Drawing for the job (mm, zero at the part's lowest x, y, z). Coordinates: 2 decimals unless noted, no trailing zeros. Write each loop counter-clockwise with the first axis right and the second up, starting at its lowest first coordinate (ties: lowest second). Pieces come first, ordered by that corner, then holes. Notation, with made-up numbers: M -14.5,-31 L 14.5,-31 A34 ccw 14.5,-1 Z; hole C 89,-5 d1. An arc over 180 degrees is marked long. Use a Markdown table: item, result. Add a question column.
Q1. Wall check: L1, parallel to Y at x = 5, z = 3; L2, parallel to X at y = 6.25, z = 1.1; L3, parallel to Z at x = 7.5, y = 4.75. Give the ranges that are in metal, low to high. Write a range as from..to.
Q2. Slice it at B-B on z = 0.8. Write the cut outline in (x, y), then the cut area to 3 significant figures.
Q3. Pin check, flat tip, straight feed: pin 1 Ø1 at (x, z) = (8, 1.5) entering from +Y. Stop position of the tip, or through.
Q4. Mould opens along X. For the marked faces 1, 2 and 3 say: released by +X, released by -X, zero draft, split by the parting line, or undercut.
Q5. Slice it at C-C on z = 4.1. Write the cut outline in (x, y).
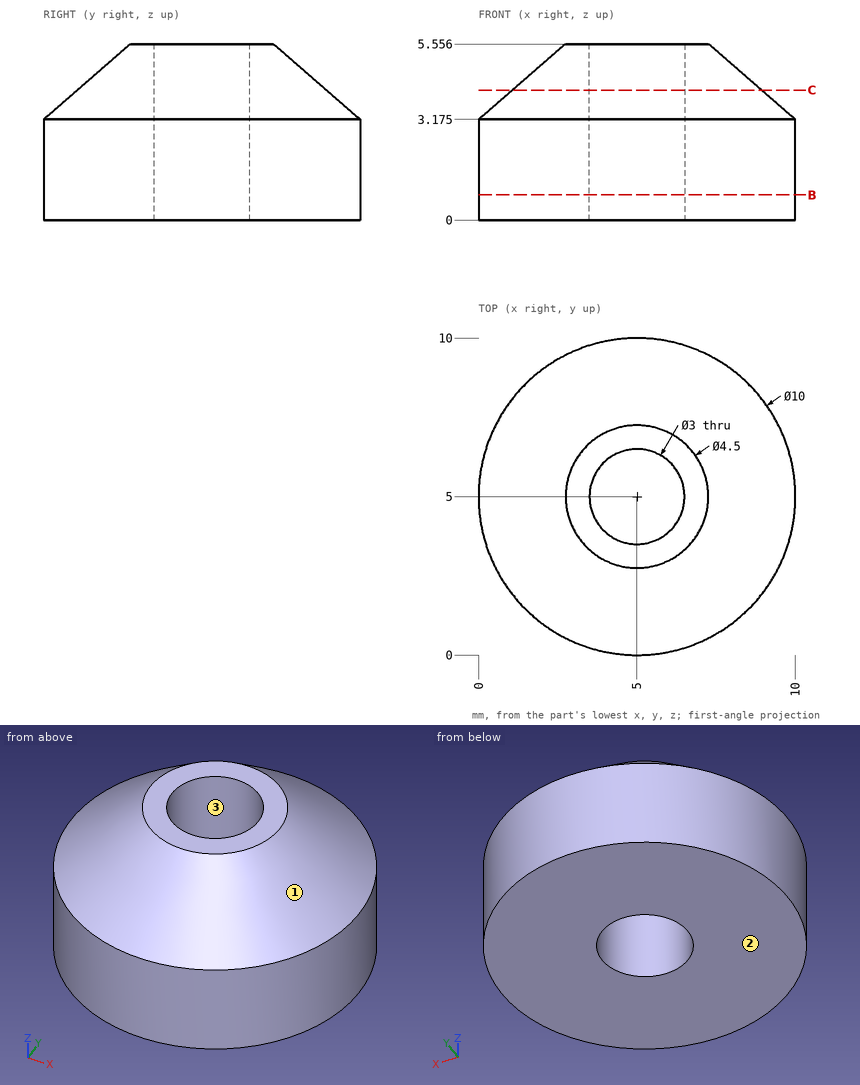
Recorded:
| question | item | result |
|---|---|---|
| 1 | L1 | 0..3.5, 6.5..10 |
| 1 | L2 | 0.16..4.17, 5.83..9.84 |
| 1 | L3 | 0..5.33 |
| 2 | outline | C 5,5 d10; hole C 5,5 d3 |
| 2 | area | 71.5 mm² |
| 3 | pin 1 | y = 9.33 |
| 4 | face 1 | split by the parting line |
| 4 | face 2 | zero draft |
| 4 | face 3 | undercut |
| 5 | outline | C 5,5 d7.86; hole C 5,5 d3 |
